Model file for the job. Use its own axes, mm. Face numbers are marked on the shaded views. A direction names the side the tool comes from. Give positions to 0.01 mm unless a question says otherwise; leave off trailing zeros. Loops run counter-clockwise (first coordinate to the right, second up) from the corner with the lowest first, then second, coordinate; pieces in that order, holes last. Notation, with made-up numbers: (73.5, -33) -> (102.5, -33) arc R21 cw to (102.5, -16) -> close; hole circle Ø4 at (75.25, 17.5). An arc over 180 degrees is marked (long way). Use CSV: the item, a comma, the result in double quotes. Start each with the question number.
(1) 3-axis set-ups, long thin cutter, end or side, ignore diameter. For the marked faces 1 and 2: which of +Z, -Z, +X, -X, +Y, -Y reach the whole face in a straight line?
(2) Drill centre lines: probe 1 along Y at (x, z) = (0, 1); probe 2 along Z at (x, y) = (3.5, 11.5); probe 3 along X at (y, z) = (-14, -17). Where is each one in solid material? Low to high.
(3) Flat gauge pins, fed straight in: pin 1 (3 mm diameter, centred on x = 12, y = -14.5, fed in from -Z); pin 2 (5 mm diameter, centred on y = -7.5, z = -17.5, fed in from +X); pin 3 (8.5 mm diameter, centred on x = 0, y = 0, fed in from -Z). Where does each tip first touch, or does it go through?
(4) Cut at C-C on z = -38.5. Write the cut outline in (x, y).
(5) Cut at B-B on y = 0. Write the cut outline in (x, z), then the cut area to 3 significant figures.
(6) Cut at D-D on y = -12.5. Write the cut outline in (x, z).
(7) Cut at A-A on x = 0. Write the cut outline in (y, z).
(8) Pull direction Y, two halves, no side cores. Call the marked faces 3, 4 and 5: pulls with the +Y half, pulls with the -Y half, needs draft (parallel to the pull), parting line crosses it, or undercut.
from build123d import *

# Parameters (mm, degrees)
SKETCH_1_W      = 50
SKETCH_1_H      = 50
SKETCH_1_R      = 7
EXTRUDE_1_DEPTH = 5
SKETCH_2_W      = 50
SKETCH_2_H      = 50
EXTRUDE_2_DEPTH = 5


with BuildPart() as part:
    # 草图1 → 凸台-拉伸1 (new body)
    with BuildSketch(Plane.XY):
        Rectangle(SKETCH_1_W, SKETCH_1_H)
        Circle(SKETCH_1_R, mode=Mode.SUBTRACT)
    extrude(amount=EXTRUDE_1_DEPTH)

    # 草图2 → 凸台-拉伸2 (add)
    with BuildSketch(Plane.ZY.offset(25)):
        with Locations((-20, 0)):
            Rectangle(SKETCH_2_W, SKETCH_2_H)
    extrude(amount=-EXTRUDE_2_DEPTH)


solid = part.part
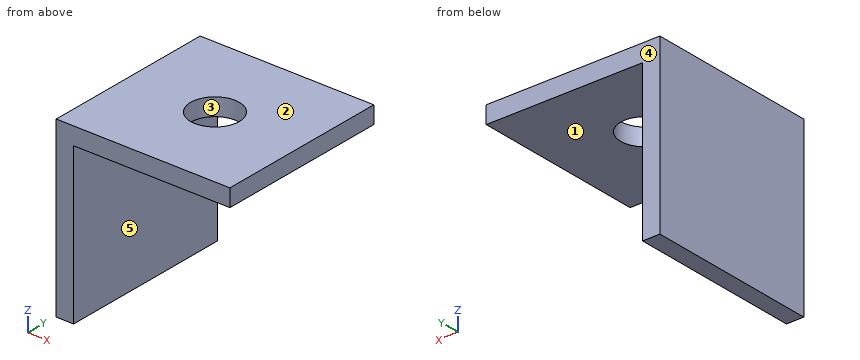
Check result:
1,face 1,"-Z, +X, +Y, -Y"
1,face 2,"+Z, +X, -X, +Y, -Y"
2,probe 1,"-25 to -7, 7 to 25"
2,probe 2,"0 to 5"
2,probe 3,"-25 to -20"
3,pin 1,"z = 0"
3,pin 2,"x = -20"
3,pin 3,"through"
4,outline,"(-25, -25) -> (-20, -25) -> (-20, 25) -> (-25, 25) -> close"
5,outline,"(-25, -45) -> (-20, -45) -> (-20, 0) -> (-7, 0) -> (-7, 5) -> (-25, 5) -> close; (7, 0) -> (25, 0) -> (25, 5) -> (7, 5) -> close"
5,area,"405 mm²"
6,outline,"(-25, -45) -> (-20, -45) -> (-20, 0) -> (25, 0) -> (25, 5) -> (-25, 5) -> close"
7,outline,"(-25, 0) -> (-7, 0) -> (-7, 5) -> (-25, 5) -> close; (7, 0) -> (25, 0) -> (25, 5) -> (7, 5) -> close"
8,face 3,"undercut"
8,face 4,"pulls with the +Y half"
8,face 5,"needs draft"
